from build123d import *

# Parameters (mm, degrees)
F0_R     = 43.165050556
F1_DEPTH = 50.8
F2_DEPTH = 12.7
F3_W     = 74.5423375242
F3_H     = 25.2622670705
F5_DEPTH = 97.5896194577
F6_DEPTH = 19.05
F7_DEPTH = 19.05
F8_DEPTH = 2.54
F9_DEPTH = 6.35


with BuildPart() as f1:
    # F0 (on Top) → F1 (new body)
    with BuildSketch(Plane.XY):
        with BuildLine():
            Line((57.0385901099, -30.2327521232), (74.4934776686, 2.6984937288))
            Line((74.4934776686, 2.6984937288), (54.7016252051, 34.2804939083))
            ThreePointArc((54.7016252051, 34.2804939083), (62.0431865669, 17.8343226196), (64.5555579534, 0))
            ThreePointArc((64.5555579534, 0), (62.6481367325, -15.5766179457), (57.0385901099, -30.2327521232))
        make_face()
        with BuildLine():
            Line((39.5837029554, -63.1639972128), (57.0385901099, -30.2327521232))
            ThreePointArc((57.0385901099, -30.2327521232), (34.280492356, -54.7016261779), (2.3369646013, -64.5132440599))
            Line((2.3369646013, -64.5132440599), (39.5837029554, -63.1639972128))
        make_face()
        with BuildLine():
            Line((-34.9097747132, -65.8624909417), (2.3369646013, -64.5132440599))
            ThreePointArc((2.3369646013, -64.5132440599), (-30.2327516987, -57.038590335), (-54.7016263939, -34.2804920112))
            Line((-54.7016263939, -34.2804920112), (-34.9097747132, -65.8624909417))
        make_face()
        with BuildLine():
            Line((-74.4934776686, -2.6984937288), (-54.7016263939, -34.2804920112))
            ThreePointArc((-54.7016263939, -34.2804920112), (-64.5132440984, -2.3369635366), (-57.0385899433, 30.2327524377))
            Line((-57.0385899433, 30.2327524377), (-74.4934776686, -2.6984937288))
        make_face()
        with BuildLine():
            ThreePointArc((2.3369646013, -64.5132440599), (34.280492356, -54.7016261779), (57.0385901099, -30.2327521232))
            ThreePointArc((57.0385901099, -30.2327521232), (62.6481367325, -15.5766179457), (64.5555579534, 0))
            ThreePointArc((64.5555579534, 0), (62.0431865669, 17.8343226196), (54.7016252051, 34.2804939083))
            ThreePointArc((54.7016252051, 34.2804939083), (30.232750983, 57.0385907143), (-2.3369639827, 64.5132440823))
            ThreePointArc((-2.3369639827, 64.5132440823), (-34.280491943, 54.7016264367), (-57.0385899433, 30.2327524377))
            ThreePointArc((-57.0385899433, 30.2327524377), (-64.5132440984, -2.3369635366), (-54.7016263939, -34.2804920112))
            ThreePointArc((-54.7016263939, -34.2804920112), (-30.2327516987, -57.038590335), (2.3369646013, -64.5132440599))
        make_face()
        Circle(F0_R, mode=Mode.SUBTRACT)
        with BuildLine():
            ThreePointArc((-57.0385899433, 30.2327524377), (-34.280491943, 54.7016264367), (-2.3369639827, 64.5132440823))
            Line((-2.3369639827, 64.5132440823), (-39.5837029554, 63.1639972128))
            Line((-39.5837029554, 63.1639972128), (-57.0385899433, 30.2327524377))
        make_face()
        with BuildLine():
            ThreePointArc((-2.3369639827, 64.5132440823), (30.232750983, 57.0385907143), (54.7016252051, 34.2804939083))
            Line((54.7016252051, 34.2804939083), (34.9097747132, 65.8624909417))
            Line((34.9097747132, 65.8624909417), (-2.3369639827, 64.5132440823))
        make_face()
        Circle(F0_R)
    extrude(amount=F1_DEPTH)

    # F0 (on Top) → F2 (cut)
    with BuildSketch(Plane.XY):
        Circle(F0_R)
    extrude(amount=F2_DEPTH, mode=Mode.SUBTRACT)

    # F3 (on face) → F5 (cut)
    with BuildSketch(Plane(origin=(-57.038590312, 30.232751742, 0), x_dir=(-0.4683214382, -0.8835581648, 0), z_dir=(-0.8835581648, 0.4683214382, 0))):
        with Locations((0, 12.7688664648)):
            Rectangle(F3_W, F3_H)
    extrude(amount=-F5_DEPTH, mode=Mode.SUBTRACT)

    # F4 (on face) → F6 (cut)
    with BuildSketch(Plane.XY):
        Polygon((14.7088014101, -43.41361173), (-10.8375270656, -44.4895269373), (-10.6687015415, -48.4980884536), (2.0200499343, -47.9636859978), (14.7088014101, -47.429283542), align=None)
        Polygon((30.3334603819, 34.3023495006), (43.9478240628, 12.8591897156), (47.7949766962, 15.3017651388), (40.9877948558, 26.0233450313), (34.1806130153, 36.7449249238), align=None)
        Polygon((44.8734362679, -9.1183725252), (33.1102969972, -31.6303372217), (37.1492056811, -33.7407814228), (43.0307753164, -22.4847990746), (48.9123449518, -11.2288167263), align=None)
    extrude(amount=F6_DEPTH, mode=Mode.SUBTRACT)

    # F4 (on face) → F7 (cut)
    with BuildSketch(Plane.XY):
        Polygon((-33.8961248298, -36.5643020277), (-30.3334603819, -34.3023495006), (-43.9478240628, -12.8591897156), (-47.5104885107, -15.1211422428), (-40.7033066702, -25.8427221352), align=None)
        Polygon((-48.6136768425, 11.0727541786), (-44.8734362679, 9.1183725252), (-33.1102969972, 31.6303372217), (-36.8505375718, 33.5847188751), (-42.7321072072, 22.3287365268), align=None)
        Polygon((-14.7088014101, 47.429283542), (-14.539975886, 43.4207220257), (11.0063525898, 44.4966372329), (10.6687015415, 48.4980884536), (-2.0200499343, 47.9636859978), align=None)
    extrude(amount=F7_DEPTH, mode=Mode.SUBTRACT)

    # F0 (on Top) + F4 (on face) → F8 (join)
    with BuildSketch(Plane.XY):
        with BuildLine():
            ThreePointArc((-57.0385899433, 30.2327524377), (-34.280491943, 54.7016264367), (-2.3369639827, 64.5132440823))
            Line((-2.3369639827, 64.5132440823), (-39.5837029554, 63.1639972128))
            Line((-39.5837029554, 63.1639972128), (-57.0385899433, 30.2327524377))
        make_face()
        with BuildLine():
            Line((-74.4934776686, -2.6984937288), (-54.7016263939, -34.2804920112))
            ThreePointArc((-54.7016263939, -34.2804920112), (-64.5132440984, -2.3369635366), (-57.0385899433, 30.2327524377))
            Line((-57.0385899433, 30.2327524377), (-74.4934776686, -2.6984937288))
        make_face()
    with BuildSketch(Plane.XY):
        with BuildLine():
            ThreePointArc((-54.7016263939, -34.2804920112), (-30.2327516987, -57.038590335), (2.3369646013, -64.5132440599))
            ThreePointArc((2.3369646013, -64.5132440599), (34.280492356, -54.7016261779), (57.0385901099, -30.2327521232))
            ThreePointArc((57.0385901099, -30.2327521232), (62.6481367325, -15.5766179457), (64.5555579534, 0))
            ThreePointArc((64.5555579534, 0), (62.0431865669, 17.8343226196), (54.7016252051, 34.2804939083))
            ThreePointArc((54.7016252051, 34.2804939083), (30.232750983, 57.0385907143), (-2.3369639827, 64.5132440823))
            ThreePointArc((-2.3369639827, 64.5132440823), (-34.280491943, 54.7016264367), (-57.0385899433, 30.2327524377))
            ThreePointArc((-57.0385899433, 30.2327524377), (-64.5132440984, -2.3369635366), (-54.7016263939, -34.2804920112))
        make_face()
        Polygon((-30.0572673127, -40.9522618745), (-27.3202242883, -39.0483151983), (-30.3334603819, -34.3023495006), (-33.8961248298, -36.5643020277), (-40.7033066702, -25.8427221352), (-47.5104885107, -15.1211422428), (-43.9478240628, -12.8591897156), (-46.7150717143, -8.5006655168), (-49.4185883118, -10.2171410057), (-54.2964744699, -2.5342779097), (-50.4943327821, 5.5542261239), (-47.4769450808, 4.1358506716), (-44.8734362679, 9.1183725252), (-48.6136768425, 11.0727541786), (-42.7321072072, 22.3287365268), (-36.8505375718, 33.5847188751), (-33.1102969972, 31.6303372217), (-30.7193281438, 36.2061060858), (-33.5575978209, 37.6891823943), (-29.342986285, 45.754987272), (-20.4370654694, 46.5064879984), (-20.1567207926, 43.1841658699), (-14.539975886, 43.4207220257), (-14.7088014101, 47.429283542), (-2.0200499343, 47.9636859978), (10.6687015415, 48.4980884536), (11.0063525898, 44.4966372329), (16.4542719722, 44.7260830931), (16.4542719722, 48.0602122843), (25.3918431699, 48.0602122843), (30.269729328, 40.3773491883), (27.5662127305, 38.6608736994), (30.3334603819, 34.3023495006), (34.1806130153, 36.7449249238), (40.9877948558, 26.0233450313), (47.7949766962, 15.3017651388), (43.9478240628, 12.8591897156), (46.9610601565, 8.1132240179), (49.8485007356, 9.7802886135), (54.3172863345, 2.0401249081), (50.1026747985, -6.0256799696), (47.2644051214, -4.542603661), (44.8734362679, -9.1183725252), (48.9123449518, -11.2288167263), (43.0307753164, -22.4847990746), (37.1492056811, -33.7407814228), (33.1102969972, -31.6303372217), (30.5067881843, -36.6128590752), (33.3942287634, -38.2799236708), (28.9254431645, -46.0200873762), (19.8329454705, -46.4030291579), (19.6981923909, -43.2034773604), (14.7088014101, -43.41361173), (14.7088014101, -47.429283542), (2.0200499343, -47.9636859978), (-10.6687015415, -48.4980884536), (-10.8375270656, -44.4895269373), (-15.9957435705, -44.7067716026), (-15.8609904909, -47.9063234), (-24.9534881849, -48.2892651817), align=None, mode=Mode.SUBTRACT)
    extrude(amount=F8_DEPTH)

    # F4 (on face) → F9 (join)
    with BuildSketch(Plane.XY):
        Polygon((27.2287273618, -42.8863195699), (19.6981923909, -43.2034773604), (19.8329454705, -46.4030291579), (28.9254431645, -46.0200873762), (33.3942287634, -38.2799236708), (30.5067881843, -36.6128590752), align=None)
        Polygon((-15.9957435705, -44.7067716026), (-23.5262785415, -45.023929393), (-27.3202242883, -39.0483151983), (-30.0572673127, -40.9522618745), (-24.9534881849, -48.2892651817), (-15.8609904909, -47.9063234), align=None)
        Polygon((-49.4185883118, -10.2171410057), (-46.7150717143, -8.5006655168), (-50.7550059033, -2.1376098231), (-47.4769450808, 4.1358506716), (-50.4943327821, 5.5542261239), (-54.2964744699, -2.5342779097), align=None)
        Polygon((-33.5575978209, 37.6891823943), (-30.7193281438, 36.2061060858), (-27.2287273618, 42.8863195699), (-20.1567207926, 43.1841658699), (-20.4370654694, 46.5064879984), (-29.342986285, 45.754987272), align=None)
        Polygon((16.4542719722, 48.0602122843), (16.4542719722, 44.7260830931), (23.5262785415, 45.023929393), (27.5662127305, 38.6608736994), (30.269729328, 40.3773491883), (25.3918431699, 48.0602122843), align=None)
        Polygon((50.7550059033, 2.1376098231), (47.2644051214, -4.542603661), (50.1026747985, -6.0256799696), (54.3172863345, 2.0401249081), (49.8485007356, 9.7802886135), (46.9610601565, 8.1132240179), align=None)
    extrude(amount=-F9_DEPTH)


solid = f1.part
Geometry: final body of the model. Coordinates: model frame, mm. A direction names the side the tool comes from. Round coordinates to 2 decimals unless told otherwise and drop trailing zeros. Loops run counter-clockwise (first coordinate to the right, second up) from the corner with the lowest first, then second, coordinate; pieces in that order, holes last.
Q1. Pin query (flat end, axial travel): P1, Ø22.5, axis at x = -11.5, y = -33.5, coming from the -Z side; P2, Ø1.4, axis at x = -1, y = -45.5, coming from the -Z side; P3, Ø1, axis at x = -41, z = 15, coming from the +Y side. Return the tip coordinate at first contact, or that it passes through.
Q2. Section B-B on x = 0. Return loops of the section in (y, z).
Q3. Material intervals for L1, parallel to Y at x = 0, z = 6.5; L2, parallel to Y at x = 8.5, z = 19; L3, parallel to X at y = -19, z = 16, sorted ascending.
Q4. Section C-C on x = 60. Return loops of the section in (y, z).
Q5. Section A-A on y = 0. Return loops of the section in (x, z), plus the area to 3 significant figures.
Q6. Access query for faces 1 (the flat face through (24.316, -46.214, -3.131)), 2 (the flat face through (23, 46, -6.35)), 3 (the flat face through (-52.4, 1.5, 1.3)), 4 (the flat face through (39.074, -20.217, 9.392)). Directions: +Z, -Z, +X, -X, +Y, -Y. A direction counts if a zero-diameter tool reaches every point of the face in a straight line with its end or side. Return the directions, or none.
Q7. Pull-direction query (X, two-part tool) for faces 5 (the flat face through (31.13, -42.2, -3.13)), 6 (the flat face through (-51, -2, -6.35)), 7 (the flat face through (-32.14, -35.45, 9.39)); classes: released by +X, released by -X, zero draft, split by the parting line, or undercut.
Evaluation:
1. P1: stops at z = 0
1. P2: stops at z = 19.05
1. P3: stops at y = -24.59
2. outline: (-64.6, 0) - (-48.05, 0) - (-48.05, 19.05) - (-44.03, 19.05) - (-44.03, 0) - (-43.17, 0) - (-43.17, 12.7) - (-42.18, 12.7) - (-42.18, 25.4) - (42.18, 25.4) - (42.18, 12.7) - (43.17, 12.7) - (43.17, 0) - (44.03, 0) - (44.03, 19.05) - (48.05, 19.05) - (48.05, 0) - (64.6, 0) - (64.6, 50.8) - (-64.6, 50.8) - close
3. L1: y = -64.6 to -48.05, -44.03 to -43.17, 43.17 to 44.03, 48.05 to 64.6
3. L2: y = -64.29 to -47.69, 37.68 to 44.39, 48.41 to 64.91
3. L3: x = -64.28 to -45.05, 27.32 to 39.71, 44.85 to 62.99
4. outline: (-24.65, 0) - (25.83, 0) - (25.83, 50.8) - (-24.65, 50.8) - close
5. outline: (-73.06, 0) - (-53.11, 0) - (-53.11, -6.35) - (-49.64, -6.35) - (-49.64, 0) - (-43.17, 0) - (-43.17, 0.14) - (-53.11, 0.14) - (-53.11, 2.54) - (-73.06, 2.54) - close; (-73.06, 25.4) - (37.39, 25.4) - (37.39, 12.7) - (43.17, 12.7) - (43.17, 0) - (49.64, 0) - (49.64, -6.35) - (53.25, -6.35) - (53.25, 0) - (73.06, 0) - (73.06, 50.8) - (-73.06, 50.8) - close
5. area: 4,640 mm2
6. face 1: -Z, +X, -Y
6. face 2: -Z, +X, -X, +Y, -Y
6. face 3: none
6. face 4: -Z
7. face 5: released by +X
7. face 6: zero draft
7. face 7: undercut
